Source: CAD feature listing. Evaluate the final solid. Frame: model axes, mm. A direction names the side the tool comes from. Give positions to 0.01 mm unless a question says otherwise; leave off trailing zeros. Order: outer loops, then holes, each group sorted by start corner. A loop starts at its lowest first (then second) coordinate and runs counter-clockwise, first axis right, second up. Notation, with made-up numbers: (49.5, 23.5) - (81.5, 23.5) arc R10 ccw to (81.5, 40.5) - close; hole circle Ø7 at (33.5, 1). An arc over 180 degrees is marked (long way). Write each question's results on one line, items separated by ' | '. Start each with the question number.
Item 1: Section D-D on z = -19.5. Output: boundary loops of the cut face in (x, y), and give its area (3 significant figures).
Item 2: Set-up query: faces 4 (the flat face through (0, -4.762, -16)), 5 (the flat face through (-3.175, 0, -16)), 6 (the flat face through (-6, 9, 0)). Return all of +Z, -Z, +X, -X, +Y, -Y with unobstructed straight access to the full face (end or side cutting, diameter ignored); none if empty.
Item 3: Section B-B on y = 0. Output: boundary loops of the cut face in (x, z) (3 decimals).
Item 4: Section A-A on x = 0. Output: boundary loops of the cut face in (y, z) (1 decimal), and give its area (3 significant figures).
Item 5: Line query: line 1 along X through (y, z) = (2.75, -19.05) (3 decimals); line 2 along Y through (x, z) = (6, -10.5). Output: solid intervals per line, ascending.
Item 6: Contact query for flat-ended pins moving along their axis: pin 1 Ø3 at (x, z) = (0, -18) entering from -Y; pin 2 Ø5 at (y, z) = (6, 5) entering from +X; pin 3 Ø14 at (x, z) = (4, -4.5) entering from +Y. Output: stop coordinate, or through.
Item 7: Section C-C on z = -2. Output: boundary loops of the cut face in (x, y).
Item 8: Mould query, pull axis X, two halves, no side actions, for faces 1 (the cylindrical face through (0.572, 0.067, -17.233)), 2 (the flat face through (12.7, 0, -6)), 3 (the flat face through (0, 12.7, -6)). Classes: released by +X, released by -X, zero draft, split by the parting line, or undercut.
```python
from build123d import *

# Parameters (mm, degrees)
SKETCH1_W           = 25.4
SKETCH1_H           = 25.4
BOSS_EXTRUDE1_DEPTH = 12.7
SKETCH3_W           = 25.4
SKETCH3_H           = 25.4
SKETCH3_R           = 10.16
CUT_EXTRUDE1_DEPTH  = 12.7
FILLET1_R           = 2.54
SKETCH4_R           = 1.905
BOSS_EXTRUDE3_DEPTH = 1.27
SKETCH5_R           = 1.905
BOSS_EXTRUDE4_DEPTH = 9.525


with BuildPart() as part:
    # Sketch1 → Boss-Extrude1 (new, symmetric)
    with BuildSketch(Plane.XY):
        Rectangle(SKETCH1_W, SKETCH1_H)
    extrude(amount=BOSS_EXTRUDE1_DEPTH, both=True)

    # Sketch3 → Cut-Extrude1 (cut)
    with BuildSketch(Plane.XY.offset(12.7)):
        Rectangle(SKETCH3_W, SKETCH3_H)
        Circle(SKETCH3_R, mode=Mode.SUBTRACT)
    extrude(amount=-CUT_EXTRUDE1_DEPTH, mode=Mode.SUBTRACT)

    # Fillet1
    fillet1_edges = [part.edges().sort_by_distance(p)[0] for p in [
        (12.7, -12.7, -6.35),
        (-12.7, -12.7, -6.35),
        (-12.7, 12.7, -6.35),
        (12.7, 12.7, -6.35),
    ]]
    fillet(fillet1_edges, radius=FILLET1_R)

    # Sketch4 → Boss-Extrude3 (add, symmetric)
    with BuildSketch(Plane(origin=(0, 12.7, 0), x_dir=(1, 0, 0), z_dir=(0, 1, 0))):
        with Locations(Location((-6.35, 8.89, 0), (0, 0, 90))):
            Circle(SKETCH4_R)
    extrude(amount=BOSS_EXTRUDE3_DEPTH, both=True)

    # Sketch5 → Boss-Extrude4 (add)
    with BuildSketch(Plane(origin=(0, 4.7625, 0), x_dir=(1, 0, 0), z_dir=(0, 1, 0))):
        with BuildLine():
            Line((-3.175, 12.7), (3.175, 12.7))
            Line((3.175, 12.7), (3.175, 19.05))
            ThreePointArc((3.175, 19.05), (0, 22.225), (-3.175, 19.05))
            Line((-3.175, 19.05), (-3.175, 12.7))
        make_face()
        with Locations(Location((0, 19.05, 0), (0, 0, 270))):
            Circle(SKETCH5_R, mode=Mode.SUBTRACT)
    extrude(amount=-BOSS_EXTRUDE4_DEPTH)


solid = part.part
```
Evaluation:
1) outline: (-3.14, -4.76) - (-1.85, -4.76) - (-1.85, 4.76) - (-3.14, 4.76) - close; (1.85, -4.76) - (3.14, -4.76) - (3.14, 4.76) - (1.85, 4.76) - close | area: 24.6 mm^2
2) face 4: -Z, +X, -X, -Y | face 5: -Z, -X, +Y, -Y | face 6: +Z
3) outline: (-12.7, -12.7) - (-3.175, -12.7) - (-3.175, -19.05) arc R3.175 ccw to (3.175, -19.05) - (3.175, -12.7) - (12.7, -12.7) - (12.7, 0) - (10.16, 0) - (10.16, 12.7) - (-10.16, 12.7) - (-10.16, 0) - (-12.7, 0) - close; hole circle Ø3.81 at (0, -19.05)
4) outline: (-12.7, -12.7) - (-4.8, -12.7) - (-4.8, -17.1) - (4.8, -17.1) - (4.8, -12.7) - (12.7, -12.7) - (12.7, 0) - (10.2, 0) - (10.2, 12.7) - (-10.2, 12.7) - (-10.2, 0) - (-12.7, 0) - close; (-4.8, -22.2) - (4.8, -22.2) - (4.8, -21) - (-4.8, -21) - close | area: 635 mm^2
5) line 1: x = -3.175 to -1.905, 1.905 to 3.175 | line 2: y = -12.7 to 12.7
6) pin 1: stops at y = -4.76 | pin 2: stops at x = 9.54 | pin 3: stops at y = 12.7
7) outline: (-12.7, -10.16) arc R2.54 ccw to (-10.16, -12.7) - (10.16, -12.7) arc R2.54 ccw to (12.7, -10.16) - (12.7, 10.16) arc R2.54 ccw to (10.16, 12.7) - (-10.16, 12.7) arc R2.54 ccw to (-12.7, 10.16) - close
8) face 1: undercut | face 2: released by +X | face 3: zero draft
